Read the model definition and answer for the solid it produces. Units are mm, in the model's axes. Round coordinates to 2 decimals unless told otherwise and drop trailing zeros. Write each loop counter-clockwise with the first axis right and the second up, starting at its lowest first coordinate (ties: lowest second). Pieces come first, ordered by that corner, then holes. Notation, with made-up numbers: (-35.5, -20.5) - (22.5, -20.5) arc R14 ccw to (22.5, 5.5) - close; hole circle Ø3 at (-2.5, 45). An arc over 180 degrees is marked (long way). One line per item, written item: value. Start each with the question number.
(1) A cutting plane is placed at B-B, the plane z = 1.35. State how many separate pieces and enclosed holes the cut face has, plus the area to 3 significant figures.
(2) A cutting plane is placed at A-A, the plane x = -24. Determine the outline of the cut face in (y, z).
(3) Find the intervals of material crossed by L1, parallel to X at y = -96, z = 3.5; L2, parallel to Y at x = -60, z = 1.35; L3, parallel to X at y = 26, z = 0.5, in increasing order.
(4) The mould has two halves that part along Y. Classify faces 1 (the face through (-77.352, -110.484, 2.465)), 2 (the face through (68.617, 64.669, 2.535)), 3 (the face through (3.75, -38.2, 2.46)): +Y half, -Y half, draft (parallel to the pull), parting line (faces both ways), or undercut.
(5) Flat-ended cylindrical pins translate along their axes: pin 1 Ø13 at (x, y) = (-60.76, -91.63) entering from -Z; pin 2 Ø9 at (x, y) = (56.82, 28.14) entering from -Z; pin 3 Ø3 at (y, z) = (-46.5, 2) entering from +X; pin 4 Ø2 at (y, z) = (24, 2) entering from +X. Find the tip coordinate at first contact, or state that the pin passes through.
from build123d import *

# Parameters (mm, degrees)
ESQUISSE1_R             = 4
BASE_EXTRUSION_DEPTH    = 5
ESQUISSE4_R             = 5
ENL_V_MAT_EXTRU_1_DEPTH = 184.114841449
ESQUISSE5_R             = 5
ENL_V_MAT_EXTRU_2_DEPTH = 5
ESQUISSE12_R            = 5
ENL_V_MAT_EXTRU_3_DEPTH = 184.114841449


with BuildPart() as part:
    # Esquisse1 → Base-Extrusion (new body)
    with BuildSketch(Plane.XY):
        with BuildLine():
            Line((75.029222277, 91.337855838), (38.048651763, 11.373375441))
            ThreePointArc((38.048651763, 11.373375441), (3.1478246, -38.807248513), (-46.811009341, -74.02482464))
            Line((-46.811009341, -74.02482464), (-123.833766756, -110.238168816))
            ThreePointArc((-123.833766756, -110.238168816), (-128.628603048, -123.542662227), (-115.324109637, -128.33749852))
            Line((-115.324109637, -128.33749852), (-38.301352222, -92.124154344))
            ThreePointArc((-38.301352222, -92.124154344), (17.334621939, -52.904580929), (56.201452189, 2.978386656))
            Line((56.201452189, 2.978386656), (93.182022703, 82.942867053))
            ThreePointArc((93.182022703, 82.942867053), (88.303116883, 96.216761659), (75.029222277, 91.337855838))
        make_face()
        with Locations((84.10562249, 87.140361446)):
            Circle(ESQUISSE1_R, mode=Mode.SUBTRACT)
    extrude(amount=BASE_EXTRUSION_DEPTH)

    # Esquisse3 → Enlèvement de matière-Révolution2 (revolve, cut)
    with BuildSketch(Plane(origin=(24.28345685, -51.648883823, 0), x_dir=(0.9049664851912627, 0.4254828559185108, 0), z_dir=(0.4254828559185108, -0.9049664851912627, 0)), mode=Mode.PRIVATE) as enl_vement_de_mati_re_r_volution2_sk:
        Polygon((-158.969859548, 5), (-153.969859548, 5), (-153.088224644, 0), (-158.969859548, 0), align=None)
    revolve(enl_vement_de_mati_re_r_volution2_sk.sketch.rotate(Axis((-119.578938197, -119.287833668, 13.424474394), (0, 0, -1)), 25.181230443), axis=Axis((-119.578938197, -119.287833668, 13.424474394), (0, 0, -1)), mode=Mode.SUBTRACT)

    # Esquisse4 → Enlèv. mat.-Extru.1 (cut, through all)
    with BuildSketch(Plane.XY.offset(5)):
        with Locations((73.611886508, 64.449360914)):
            Circle(ESQUISSE4_R)
        with Locations((65.216897723, 46.296560488)):
            Circle(ESQUISSE4_R)
        with Locations((56.821908937, 28.143760062)):
            Circle(ESQUISSE4_R)
        with Locations((48.426920152, 9.990959637)):
            Circle(ESQUISSE4_R)
        with Locations((40.031931366, -8.161840789)):
            Circle(ESQUISSE4_R)
    extrude(amount=-ENL_V_MAT_EXTRU_1_DEPTH, mode=Mode.SUBTRACT)

    # Esquisse5 → Enlèv. mat.-Extru.2 (cut)
    with BuildSketch(Plane.XY.offset(5)):
        with Locations((-96.954776067, -108.65076227)):
            Circle(ESQUISSE5_R)
        with Locations((-78.855446363, -100.141105152)):
            Circle(ESQUISSE5_R)
        with Locations((-60.756116659, -91.631448033)):
            Circle(ESQUISSE5_R)
        with Locations((-42.656786955, -83.121790915)):
            Circle(ESQUISSE5_R)
        with Locations((-24.557457251, -74.612133797)):
            Circle(ESQUISSE5_R)
    extrude(amount=-ENL_V_MAT_EXTRU_2_DEPTH, mode=Mode.SUBTRACT)

    # Esquisse12 → Enlèv. mat.-Extru.3 (cut, through all)
    with BuildSketch(Plane.XY.offset(5)):
        with Locations((-1.909251541, -58.652301466)):
            Circle(ESQUISSE12_R)
        with Locations((14.143088399, -43.608286628)):
            Circle(ESQUISSE12_R)
        with Locations((28.319996864, -26.785229047)):
            Circle(ESQUISSE12_R)
    extrude(amount=-ENL_V_MAT_EXTRU_3_DEPTH, mode=Mode.SUBTRACT)


solid = part.part
Here are the results:
1. separate pieces: 1
1. enclosed holes: 15
1. area: 5,200 mm²
2. outline: (-84.67, 0) - (-79.58, 0) - (-79.58, 5) - (-84.67, 5) - close; (-69.64, 0) - (-61.15, 0) - (-61.15, 5) - (-69.64, 5) - close
3. L1: -93.55 to -81.66, -76.05 to -63.19, -58.32 to -46.54
3. L2: -102.33 to -96.57, -86.69 to -80.23
3. L3: 44.81 to 52.3, 61.34 to 66.85
4. face 1: -Y half
4. face 2: undercut
4. face 3: +Y half
5. pin 1: z = 0
5. pin 2: through
5. pin 3: x = 24.77
5. pin 4: x = 66.39
